from build123d import *

# Parameters (mm, degrees)
F0_W     = 956
F0_H     = 396
F1_DEPTH = 146
F2_T     = -22
F3_R     = 11
F4_R     = 11


with BuildPart() as f1:
    # F0 (on Front) → F1 (new body)
    with BuildSketch(Plane.XZ):
        Rectangle(F0_W, F0_H)
    extrude(amount=F1_DEPTH)

    # F2
    f2_openings = [f1.faces().sort_by_distance(p)[0] for p in [
        (0, -146, 0),
    ]]
    offset(amount=F2_T, openings=f2_openings)

    # F3
    f3_edges = [f1.edges().sort_by_distance(p)[0] for p in [
        (-478, -73, -198),
        (478, -73, -198),
        (0, 0, -198),
        (0, -146, -198),
    ]]
    fillet(f3_edges, radius=F3_R)

    # F4
    f4_edges = [f1.edges().sort_by_distance(p)[0] for p in [
        (478, -73, 198),
        (-478, -73, 198),
        (0, 0, 198),
        (0, -146, 198),
    ]]
    fillet(f4_edges, radius=F4_R)


solid = f1.part
The model under review builds one solid part; all positions refer to its coordinate system, in mm. A direction names the side the tool comes from. Coordinates: 2 decimals unless noted, no trailing zeros. Write each loop counter-clockwise with the first axis right and the second up, starting at its lowest first coordinate (ties: lowest second). Pieces come first, ordered by that corner, then holes. Notation, with made-up numbers: (35, 41.25) - (90, 41.25) arc R24 cw to (90, 79.25) - close; hole circle Ø6 at (88, 46.25). An arc over 180 degrees is marked (long way). Answer as a JSON object with one key per item and string values. Group by question number.
1. Add section C-C (x = -96). Give the boundary of the cut face in (y, z), plus the area to 3 significant figures.
2. Add section A-A (y = -110). Give the boundary of the cut face in (x, z).
3. Add section B-B (z = -108). Give the boundary of the cut face in (x, y).
4. Machinability: for faces 1 (the face through (456, -83, -2)), 2 (the face through (478, -72, -3)), which of the approach directions +Z, -Z, +X, -X, +Y, -Y give a long, thin tool a straight path to every point of the face, cutting with its end or side? Answer none if there is none.
5. Mouldability with a two-part tool opening along Z and no side actions: class faces 3 (the face through (-6, -83, 176)), 4 (the face through (-6, -22, 2)), 5 (the face through (-7, -72, -198)), 6 (the face through (-478, -72, -3)) as pulls with the +Z half, pulls with the -Z half, needs draft (parallel to the pull), parting line crosses it, or undercut.
6. To check wall thickness, follow probe 1 along Z at (x, y) = (197, -81.5); probe 2 along X at (y, z) = (-139, 64); probe 3 along Y at (x, z) = (405, 112.5). State the ranges of each line that lie inside material, in increasing order.
Findings:
{
 "1": {"outline": "(-146, -187) arc R11 ccw to (-135, -198) - (-11, -198) arc R11 ccw to (0, -187) - (0, 187) arc R11 ccw to (-11, 198) - (-135, 198) arc R11 ccw to (-146, 187) - (-146, 176) - (-22, 176) - (-22, -176) - (-146, -176) - close", "area": "14,100 mm²"},
 "2": {"outline": "(-478, -187) arc R11 ccw to (-467, -198) - (467, -198) arc R11 ccw to (478, -187) - (478, 187) arc R11 ccw to (467, 198) - (-467, 198) arc R11 ccw to (-478, 187) - close; hole (-456, -176) - (456, -176) - (456, 176) - (-456, 176) - close"},
 "3": {"outline": "(-478, -146) - (-456, -146) - (-456, -22) - (456, -22) - (456, -146) - (478, -146) - (478, 0) - (-478, 0) - close"},
 "4": {"face 1": "-Y", "face 2": "+Z, -Z, +X, +Y, -Y"},
 "5": {"face 3": "undercut", "face 4": "undercut", "face 5": "pulls with the -Z half", "face 6": "needs draft"},
 "6": {"probe 1": "-198 to -176, 176 to 198", "probe 2": "-478 to -456, 456 to 478", "probe 3": "-22 to 0"}
}
